Model file for the job. Use its own axes, mm. A direction names the side the tool comes from. Round coordinates to 2 decimals unless told otherwise and drop trailing zeros. Loops run counter-clockwise (first coordinate to the right, second up) from the corner with the lowest first, then second, coordinate; pieces in that order, holes last.
from build123d import *

# Parameters (mm, degrees)
BASIS_BLECH1_DEPTH                   = 45
SKIZZE3_R                            = 5
SCHNITT_LINEAR_AUSTRAGEN2_DEPTH      = 67.708320321
SCHNITT_LINEAR_AUSTRAGEN1_DEPTH      = 67.708320321
SCHNITT_LINEAR_AUSTRAGEN1_DEPTH_BACK = 67.708320321
F_3_0_3_DURCHMESSER_BOHRUNG1_D       = 3
F_3_0_3_DURCHMESSER_BOHRUNG2_D       = 3


# Sheet-metal steps are written as plain solids
with BuildPart() as part:
    # Skizze1 → Basis-Blech1 (new, symmetric)
    with BuildSketch(Plane.XY):
        with BuildLine():
            Line((-17, 45), (-17, 5))
            ThreePointArc((-17, 5), (-15.535533906, 1.464466094), (-12, 0))
            Line((-12, 0), (12, 0))
            ThreePointArc((12, 0), (15.535533906, 1.464466094), (17, 5))
            Line((17, 5), (17, 45))
            Line((17, 45), (20, 45))
            Line((20, 45), (20, 5))
            ThreePointArc((20, 5), (17.656854249, -0.656854249), (12, -3))
            Line((12, -3), (-12, -3))
            ThreePointArc((-12, -3), (-17.656854249, -0.656854249), (-20, 5))
            Line((-20, 5), (-20, 45))
            Line((-20, 45), (-17, 45))
        make_face()
    extrude(amount=BASIS_BLECH1_DEPTH, both=True)

    # Skizze3 → Schnitt-Linear austragen2 (cut, through all)
    with BuildSketch(Plane(origin=(0, 0, 0), x_dir=(1, 0, 0), z_dir=(0, 1, 0))):
        with Locations(Location((0, -30, 0), (0, 0, 270))):
            Circle(SKIZZE3_R)
    extrude(amount=-SCHNITT_LINEAR_AUSTRAGEN2_DEPTH, mode=Mode.SUBTRACT)

    # Skizze2 → Schnitt-Linear austragen1 (cut, two sides: drawn at the far end of the back side and taken through both)
    with BuildSketch(Plane(origin=(0, 0, 0), x_dir=(0, 0, -1), z_dir=(1, 0, 0)).offset(-SCHNITT_LINEAR_AUSTRAGEN1_DEPTH_BACK)):
        with BuildLine():
            Line((35, 45), (5, 45))
            Line((5, 45), (5, 20))
            ThreePointArc((5, 20), (6.464466094, 16.464466094), (10, 15))
            Line((10, 15), (30, 15))
            ThreePointArc((30, 15), (33.535533906, 16.464466094), (35, 20))
            Line((35, 20), (35, 45))
        make_face()
        Polygon((-45, 45), (-5, 45), (-45, 17), align=None)
        Polygon((45, 45), (40, 45), (45, 35), align=None)
        with BuildLine():
            Line((-5, 29.472788823), (-5, 14))
            ThreePointArc((-5, 14), (-5.878679656, 11.878679656), (-8, 11))
            Line((-8, 11), (-30.103984032, 11))
            ThreePointArc((-30.103984032, 11), (-32.965197698, 13.098081845), (-31.824371066, 16.457695762))
            Line((-31.824371066, 16.457695762), (-9.720387033, 31.930484584))
            ThreePointArc((-9.720387033, 31.930484584), (-6.614568858, 32.133724852), (-5, 29.472788823))
        make_face()
    extrude(amount=SCHNITT_LINEAR_AUSTRAGEN1_DEPTH + SCHNITT_LINEAR_AUSTRAGEN1_DEPTH_BACK, mode=Mode.SUBTRACT)

    # Ø3.0 (3) Durchmesser Bohrung1 (through all)
    with Locations(Plane.ZY.offset(20)):
        with Locations((-37.3, 39.5), (-37.3, 17.5), (-31, 12.2), (-9, 12.2), (-2.7, 17.5), (-2.7, 39.5)):
            Hole(F_3_0_3_DURCHMESSER_BOHRUNG1_D / 2)

    # Ø3.0 (3) Durchmesser Bohrung2 (through all)
    with Locations(Plane(origin=(0, 0, 0), x_dir=(1, 0, 0), z_dir=(0, 1, 0))):
        with Locations((10.162674858, -25.790482244), (4.209517756, -19.837325142), (-4.209517756, -19.837325142), (-10.162674858, -25.790482244), (-10.162674858, -34.209517756), (-4.209517756, -40.162674858), (4.209517756, -40.162674858), (10.162674858, -34.209517756)):
            Hole(F_3_0_3_DURCHMESSER_BOHRUNG2_D / 2)


solid = part.part
Q1. Pull direction Y, two halves, no side cores. Call faces 6 (the face through (0, -3, 1)), 7 (the face through (18.479, 24.086, 20.927)), 8 (the face through (18, 45, -37)): pulls with the +Y half, pulls with the -Y half, needs draft (parallel to the pull), parting line crosses it, or undercut.
Q2. Flat gauge pins, fed straight in: P1, Ø2.5, axis at x = -10.16, z = 34.21, coming from the -Y side; P2, Ø3.5, axis at x = -4.21, z = 19.84, coming from the +Y side; P3, Ø1.5, axis at x = -18.5, y = 38, coming from the -Z side (3 decimals); P4, Ø3.5, axis at x = -18, y = 27, coming from the +Z side. Where does each tip first touch, or does it go through?
Q3. Probe line 1 (X direction, y = 9, z = 20); line 2 (Y direction, x = 18, z = -2); line 3 (Y direction, x = 8.5, z = 13). List the from-to ranges inside material, lowest first.
Q4. Slice it at A-A on z = -37.3. Give the cut face in (x, y), plus the area to 3 significant figures.
Q5. Slice it at C-C on y = 39.5. State how many separate pieces and enclosed holes the cut face has, plus the area to 3 significant figures.
Q6. Slice it at D-D on z = -9. Give the cut face in (x, y).
Q7. Tool access for faces 1 (the face through (18, 17, -6)), 2 (the face through (-19, 22, 5)), 3 (the face through (18, 45, 0)), 4 (the face through (-17, 21, 1)), 5 (the face through (4.535, -1.521, 21.302)): list every direction of +Z, -Z, +X, -X, +Y, -Y with a clear straight run to the whole face (end or side of a thin tool).
Q8. Slice it at B-B on x = 0. Give the cut face in (y, z), plus the area to 3 significant figures.
Reply:
1. face 6: pulls with the -Y half
1. face 7: undercut
1. face 8: pulls with the +Y half
2. P1: passes through
2. P2: stops at y = 0
2. P3: stops at z = -43.875
2. P4: stops at z = 33.21
3. line 1: x = -20 to -17, 17 to 20
3. line 2: y = -0.29 to 16.17, 18.83 to 38.17, 40.83 to 45
3. line 3: y = -3 to 0
4. outline: (-20, 5) arc R8 ccw to (-12, -3) - (12, -3) arc R8 ccw to (20, 5) - (20, 16) - (17, 16) - (17, 5) arc R5 cw to (12, 0) - (-12, 0) arc R5 cw to (-17, 5) - (-17, 16) - (-20, 16) - close; (-20, 19) - (-17, 19) - (-17, 38) - (-20, 38) - close; (-20, 41) - (-17, 41) - (-17, 45) - (-20, 45) - close; (17, 19) - (20, 19) - (20, 38) - (17, 38) - close; (17, 41) - (20, 41) - (20, 45) - (17, 45) - close
4. area: 337 mm2
5. separate pieces: 8
5. enclosed holes: 0
5. area: 118 mm2
6. outline: (-20, 5) arc R8 ccw to (-12, -3) - (12, -3) arc R8 ccw to (20, 5) - (20, 10.7) - (17, 10.7) - (17, 5) arc R5 cw to (12, 0) - (-12, 0) arc R5 cw to (-17, 5) - (-17, 10.7) - (-20, 10.7) - close; (-20, 13.7) - (-17, 13.7) - (-17, 15.1) - (-20, 15.1) - close; (17, 13.7) - (20, 13.7) - (20, 15.1) - (17, 15.1) - close
7. face 1: +X, -X, +Y
7. face 2: +X, -X
7. face 3: +Z, -Z, +X, -X, +Y
7. face 4: +Z, -Z, +Y
7. face 5: +Y, -Y
8. outline: (-3, -45) - (0, -45) - (0, 25) - (-3, 25) - close; (-3, 35) - (0, 35) - (0, 45) - (-3, 45) - close
8. area: 240 mm2
